Geometry check sheet. Reference: the model listing, model coordinates, mm. Face numbers are marked on the shaded views. A direction names the side the tool comes from. Round coordinates to 2 decimals unless told otherwise and drop trailing zeros. Write each loop counter-clockwise with the first axis right and the second up, starting at its lowest first coordinate (ties: lowest second). Pieces come first, ordered by that corner, then holes. Notation, with made-up numbers: (30, 28.25) - (77, 28.25) arc R26 ccw to (77, 42.25) - close; hole circle Ø3 at (18.25, -18). An arc over 180 degrees is marked (long way). Return JSON: item names as keys, results as strings. Group by question number.
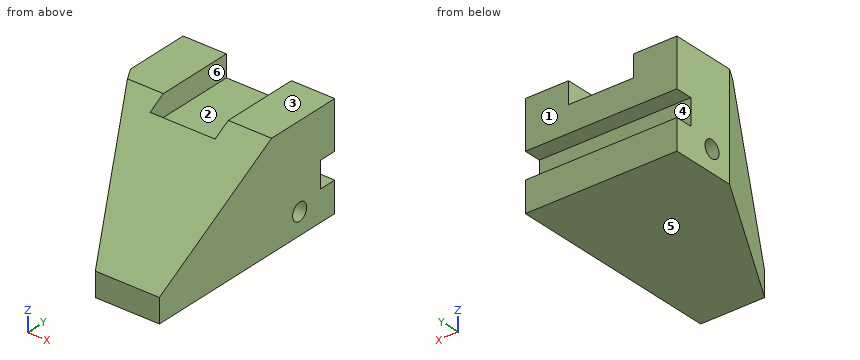
from build123d import *

# Parameters (mm, degrees)
F1_DEPTH = 120
F3_DEPTH = 175.001
F4_W     = 75
F4_H     = 108.811668
F5_DEPTH = 25
F6_W     = 20
F6_H     = 30
F6_R     = 10
F7_DEPTH = 175.001


with BuildPart() as f1:
    # F0 (on Top) → F1 (new body)
    with BuildSketch(Plane.XY):
        Polygon((-29.908918, 96.077366), (-79.908918, 96.077366), (-79.908918, 21.077366), (21.127379, -153.922634), (95.091082, -153.922634), (95.091082, 96.077366), (32.76388, 96.077366), align=None)
    extrude(amount=F1_DEPTH)

    # F2 (on face) → F3 (cut, through all)
    with BuildSketch(Plane.YZ.offset(95.091082)):
        Polygon((-153.922634, 27.623957), (6.077366, 120), (-153.922634, 120), align=None)
    extrude(amount=-F3_DEPTH, mode=Mode.SUBTRACT)

    # F4 (on face) → F5 (cut)
    with BuildSketch(Plane.XY.offset(120)):
        with Locations((7.591082, 41.671532)):
            Rectangle(F4_W, F4_H)
    extrude(amount=-F5_DEPTH, mode=Mode.SUBTRACT)

    # F6 (on face) → F7 (cut, through all)
    with BuildSketch(Plane(origin=(-79.908918, 0, 0), x_dir=(0, -1, 0), z_dir=(-1, 0, 0))):
        with Locations((-86.077366, 50)):
            Rectangle(F6_W, F6_H)
        with Locations((-46.077366, 25)):
            Circle(F6_R)
    extrude(amount=-F7_DEPTH, mode=Mode.SUBTRACT)


solid = f1.part
1. Material ranges on line 1 along X through (y, z) = (73.5, 112.5); line 2 along Y through (x, z) = (-38.5, 26); line 3 along Z through (x, y) = (33.5, 47.5), recorded low to high.
2. Depth check by flat-ended pin: pin 1 Ø7 at (x, z) = (7, 101.5) entering from +Y; pin 2 Ø10 at (y, z) = (-125, 40.5) entering from -X; pin 3 Ø22 at (x, y) = (33, 87) entering from +Z. Enter the tip coordinate at first touch or a pass-through.
3. Mould release check, pull along Z, two halves, no side actions. Record for the marked faces 3, 4, 5 and 6: pulls with the +Z half, pulls with the -Z half, needs draft (parallel to the pull), parting line crosses it, or undercut.
4. Section check B-B (z = 25). Enter the section's corners in (x, y).
5. Section check A-A (x = 57). Enter the section's corners in (y, z).
6. Section check C-C (y = -8.5). Enter the section's corners in (x, z), and give its area (3 significant figures).
7. Tool access check on the marked faces 1 and 2. Record the directions out of +Z, -Z, +X, -X, +Y, -Y that give a thin tool (end or side, any length) a straight path to the whole face; none if there is none.
8. Section check D-D (x = -68.5). Enter the section's corners in (y, z), and give its area (3 significant figures).
Result sheet:
{
 "1": {"line 1": "x = -79.91 to -29.91, 45.09 to 95.09", "line 2": "y = -50.64 to 36.13, 56.03 to 96.08", "line 3": "z = 0 to 15.1, 34.9 to 95"},
 "2": {"pin 1": "stops at y = -12.73", "pin 2": "stops at x = 1.54", "pin 3": "stops at z = 95"},
 "3": {"face 3": "pulls with the +Z half", "face 4": "undercut", "face 5": "pulls with the -Z half", "face 6": "needs draft"},
 "4": {"outline": "(-79.91, 21.08) - (21.13, -153.92) - (95.09, -153.92) - (95.09, 36.08) - (-79.91, 36.08) - close; (-79.91, 56.08) - (95.09, 56.08) - (95.09, 96.08) - (-79.91, 96.08) - close"},
 "5": {"outline": "(-153.92, 0) - (96.08, 0) - (96.08, 35) - (76.08, 35) - (76.08, 65) - (96.08, 65) - (96.08, 120) - (6.08, 120) - (-153.92, 27.62) - close; hole circle Ø20 at (46.08, 25)"},
 "6": {"outline": "(-62.83, 0) - (95.09, 0) - (95.09, 111.58) - (45.09, 111.58) - (45.09, 95) - (-29.91, 95) - (-29.91, 111.58) - (-62.83, 111.58) - close", "area": "16,400 mm²"},
 "7": {"face 1": "+Z, -Z, +X, -X, +Y", "face 2": "+Z, +Y"},
 "8": {"outline": "(1.32, 0) - (96.08, 0) - (96.08, 35) - (76.08, 35) - (76.08, 65) - (96.08, 65) - (96.08, 120) - (6.08, 120) - (1.32, 117.25) - close; hole circle Ø20 at (46.08, 25)", "area": "10,500 mm²"}
}
